Geometry check sheet. Reference: the model listing, model coordinates, mm. Face numbers are marked on the shaded views. Give positions to 0.01 mm unless a question says otherwise; leave off trailing zeros. Order: outer loops, then holes, each group sorted by start corner. A loop starts at its lowest first (then second) coordinate and runs counter-clockwise, first axis right, second up.
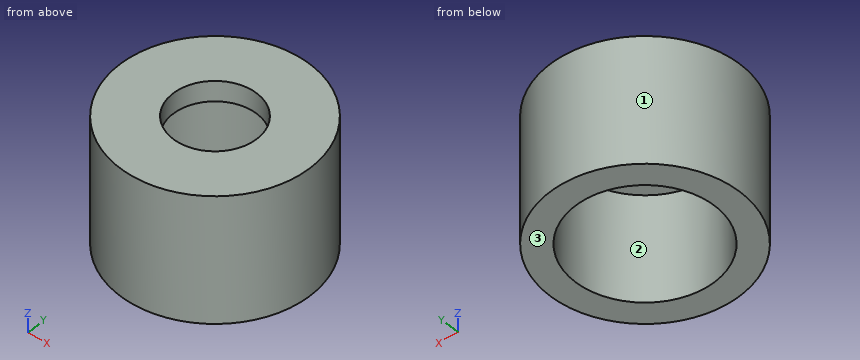
from build123d import *

# Parameters (mm, degrees)
SZKIC1_W                    = 10
SZKIC1_H                    = 7.5
SZKIC3_R                    = 5.625
DODANIE_WYCI_GNI_CIE1_DEPTH = 3.75


with BuildPart() as part:
    # Szkic1 → Obrót1 (revolve)
    with BuildSketch(Plane(origin=(0, 0, 0), x_dir=(0, 0, -1), z_dir=(1, 0, 0)), mode=Mode.PRIVATE) as obr_t1_sk:
        with Locations((-5, 3.75)):
            Rectangle(SZKIC1_W, SZKIC1_H)
    revolve(obr_t1_sk.sketch.rotate(Axis((0, 0, 0), (0, 0, 1)), 270), axis=Axis((0, 0, 0), (0, 0, 1)))

    # Szkic2 → Wycięcie-obrót1 (revolve, cut)
    with BuildSketch(Plane(origin=(0, 0, 0), x_dir=(0, 0, -1), z_dir=(1, 0, 0)), mode=Mode.PRIVATE) as wyci_cie_obr_t1_sk:
        Polygon((-10, 0), (-10, 3.3), (-8.4, 3.3), (-8.4, 5.5), (0, 5.5), (0, 0), align=None)
    revolve(wyci_cie_obr_t1_sk.sketch.rotate(Axis((0, 0, 0), (0, 0, 1)), 270), axis=Axis((0, 0, 0), (0, 0, 1)), mode=Mode.SUBTRACT)


with BuildPart() as body_2:
    # Szkic3 → Dodanie-wyciągnięcie1 (new body)
    with BuildSketch(Plane(origin=(0, 0, 0), x_dir=(0, 0, -1), z_dir=(1, 0, 0))):
        Circle(SZKIC3_R)
    extrude(amount=DODANIE_WYCI_GNI_CIE1_DEPTH)

    # Usuń ścianę1: 1 face struck out; the rest of the skin is kept as a surface, the solid goes
    usu_cian_1_1_drop = [body_2.part.faces().sort_by_distance(Vector(p))[0] for p in ((3.75, 0, 0),)]
    usu_cian_1_1 = Shell(body_2.part.faces() - usu_cian_1_1_drop)


solid = part.part
Item 1: Scan lines: L1, parallel to Y at x = 0, z = 4.75; L2, parallel to Y at x = 0, z = 9.2; L3, parallel to X at y = -0.5, z = 2.5. Record each from-to range of solid material in increasing order.
Reported:
L1: y = -7.5 to -5.5, 5.5 to 7.5
L2: y = -7.5 to -3.3, 3.3 to 7.5
L3: x = -7.48 to -5.48, 5.48 to 7.48
Item 2: Gauge pin test, flat ends, axial feed: pin 1 (5 mm diameter, centred on x = 3, z = 9, fed in from +Y); pin 2 (2 mm diameter, centred on x = 4.5, z = 6, fed in from -Y); pin 3 (4 mm diameter, centred on x = 3, z = 1.5, fed in from +Y). Record the tip position at first contact, or that the pin passes through.
Reported:
pin 1: stops at y = 7.48
pin 2: stops at y = -6.63
pin 3: stops at y = 7.43
Item 3: Draft check along X on the marked faces 1, 2 and 3. Enter one of: released by +X, released by -X, zero draft, split by the parting line, or undercut.
Reported:
face 1: split by the parting line
face 2: undercut
face 3: zero draft
Item 4: Sectioned sample at A-A (x = 0). Enter the section's corners in (y, z), and give its area (3 significant figures).
Reported:
outline: (-7.5, 0) - (-5.5, 0) - (-5.5, 8.4) - (-3.3, 8.4) - (-3.3, 10) - (-7.5, 10) - close; (3.3, 8.4) - (5.5, 8.4) - (5.5, 0) - (7.5, 0) - (7.5, 10) - (3.3, 10) - close
area: 47.0 mm2
Item 5: Sectioned sample at C-C (z = 8.75). Enter the section's corners in (x, y), and give its area (3 significant figures).
Reported:
outline: circle Ø15 at (0, 0); hole circle Ø6.6 at (0, 0)
area: 143 mm2
Item 6: Sectioned sample at D-D (y = 5). Enter the section's corners in (x, z).
Reported:
outline: (-5.59, 0) - (-2.29, 0) - (-2.29, 8.4) - (2.29, 8.4) - (2.29, 0) - (5.59, 0) - (5.59, 10) - (-5.59, 10) - close
